The listing builds one solid part. Answer for the finished solid, in the listing's coordinates (mm). A direction names the side the tool comes from. Round coordinates to 2 decimals unless told otherwise and drop trailing zeros. Order: outer loops, then holes, each group sorted by start corner. A loop starts at its lowest first (then second) coordinate and runs counter-clockwise, first axis right, second up. Notation, with made-up numbers: (60, 32) - (70, 32) arc R9 cw to (70, 43) - close; hole circle Ø4 at (-21.75, 1). An arc over 180 degrees is marked (long way). One line per item, written item: value. Start each with the question number.
1. Flat-ended cylindrical pins translate along their axes: P1, Ø2, axis at x = 61.5, z = 25.5, coming from the +Y side; P2, Ø3, axis at x = 27.5, z = -29, coming from the -Y side; P3, Ø12, axis at x = 96.5, z = -0.5, coming from the +Y side; P4, Ø2.5, axis at x = 73, z = 32.689, coming from the -Y side. Find the tip coordinate at first contact, or state that the pin passes through.
2. Section D-D, the plane x = 109 is taken. Give the vertices of the cut face in (y, z), then the cut area to 3 significant figures.
3. Section C-C, the plane z = -16 is taken. Give the vertices of the cut face in (x, y), then the cut area to 3 significant figures.
4. A tool of negligible diameter and unlimited length cuts with its end or side. For faces 4 (the flat face through (44, -23, -7.451)), 5 (the flat face through (44, -25, 17.689)), 6 (the flat face through (63, -21, -10.131)), from which of +Z, -Z, +X, -X, +Y, -Y can it reach the whole face along a straight path? Write none if from no direction.
5. Section B-B, the plane x = 73 is taken. Count the separate pieces of the cut face and the enclosed holes in it, then the cut area to 3 significant figures.
6. Straight lines are drawn through the part: line 1 (Z direction, x = 73, y = -25); line 2 (X direction, y = -24, z = -31); line 3 (Z direction, x = 37, y = -4). For each, find the intervals that lie inside material, in ascending order.
7. For a pull along X with two mould halves and no side action, classify faces 1 (the flat face through (18, -3, -26)), 2 (the flat face through (97.72, -9.847, 20.896)), 3 (the cylindrical face through (62.86, -16.74, 20.36)) as released by +X, released by -X, zero draft, split by the parting line, or undercut.
Autodesk Inventor part; units mm, degrees
ref_plane "YZ Plane" through (0, 0, 0) normal (1, 0, 0) x (0, 1, 0)
ref_plane "XZ Plane" through (0, 0, 0) normal (0, 1, 0) x (-1, 0, 0)
ref_plane "XY Plane" through (0, 0, 0) normal (0, 0, 1) x (1, 0, 0)
ref_plane "Plan de construction16" through (10, -26.1714, -17.6889) normal (0, -1, 0) x (1, 0, 0)
sketch "Esquisse9" plane through (10, -26.1714, -17.6889) normal (0, -1, 0) x (1, 0, 0)
  line L0 (0, 35.3779) -> (8, 35.3779)
  line L1 (68, 1.8848) -> (68, 33.493)
  line L2 (0, 35.3779) -> (68, 35.3779)
  line L3 (68, 35.3779) -> (68, 32.0585)
  line L4 (0, 32.0585) -> (0, 35.3779)
  line L5 (0, 0) -> (8, 0)
  line L6 (0, 37.6889) -> (0, -2.3111)
  line L7 (68, 0) -> (0, 0)
  line L8 (0, 0) -> (0, 3.3237)
  line L9 (68, 3.3237) -> (68, 0)
  line L10 (68, 35.3779) -> (0, 35.3779)
  line L11 (0, 35.3779) -> (0, 0)
  line L12 (0, 0) -> (68, 0)
  line L13 (68, 0) -> (68, 35.3779)
  point P0 (-10, 17.6889)
  point P1 (67.75, 35.3779)
  point P2 (67.75, 0)
extrude "Extrusion11" add sketch "Esquisse9" against normal blind 3
ref_plane "Plan de construction18" through (78, -26.1714, -17.6889) normal (0, -1, 0) x (1, 0, 0)
sketch "Esquisse13" plane through (78, -26.1714, -17.6889) normal (0, -1, 0) x (1, 0, 0)
  line L0 (-65, 35.3779) -> (-60, 35.3779)
  line L1 (0, 35.3779) -> (-10, 35.3779)
  line L2 (-10, 35.3779) -> (-10, 55.3779)
  line L3 (-10, 55.3779) -> (0, 55.3779)
  line L4 (0, 55.3779) -> (0, 35.3779)
  line L5 (0, 35.3779) -> (0, 0) construction
  line L6 (0, 17.6889) -> (-68.1792, 17.6889) construction
  line L7 (-68.1792, 35.3779) -> (-58.1792, 35.3779)
  line L8 (-58.1792, 35.3779) -> (-58.1792, 55.3779)
  line L9 (-58.1792, 55.3779) -> (-68.1792, 55.3779)
  line L10 (-68.1792, 55.3779) -> (-68.1792, 35.3779)
  line L11 (-65, 0) -> (0, 0)
  line L12 (0, 0) -> (-10, 0)
  line L13 (-10, 0) -> (-10, -20)
  line L14 (-10, -20) -> (0, -20)
  line L15 (0, -20) -> (0, 0)
  line L16 (-68.1792, 0) -> (-58.1792, 0)
  line L17 (-58.1792, 0) -> (-58.1792, -20)
  line L18 (-58.1792, -20) -> (-68.1792, -20)
  line L19 (-68.1792, -20) -> (-68.1792, 0)
  line L20 (-5, 34.0863) -> (-5, 43.2092) construction
  circle A0 centre (-5, 50.3779) radius 2.25
  circle A1 centre (-63.1792, 50.3779) radius 2.25
  circle A2 centre (-63.1792, -15) radius 2.25
  line L21 (-5, -1.4113) -> (-5, -11.1612)
  circle A3 centre (-5, -15) radius 2.25
  point P0 (-78, 17.6889)
  point P1 (0, 1.8848)
  point P2 (0, 33.493)
  point P3 (-0.25, 35.3779)
  dimension "d45" = 10
  dimension "d46" = 20
  dimension "d47" = 10
  dimension "d48" = 20
  dimension "d49" = 4.5
  dimension "d50" = 4.5
  dimension "d51" = 4.5
  dimension "d52" = 4.5
  dimension "d57" = 0
  dimension "d58" = 5
  dimension "d59" = 5
  dimension "d60" = 5
  dimension "d61" = 5
extrude "Extrusion12" add sketch "Esquisse13" against normal blind 3
ref_plane "Plan de construction19" through (18, 0, 0) normal (1, 0, 0) x (0, 0, -1)
sketch "Esquisse14" plane through (18, 0, 0) normal (1, 0, 0) x (0, 0, -1)
  line L0 (-19.134, -23.1714) -> (-15.8041, -23.1714)
  line L1 (-19.134, -23.1714) -> (-15.8041, -23.1714)
  line L2 (-15.8041, -23.1714) -> (-36.599, 20)
  line L3 (-38.4838, 17) -> (-19.134, -23.1714)
  line L4 (-19.134, -23.1714) -> (-15.8041, -23.1714)
  line L5 (-19.134, -23.1714) -> (-15.8041, -23.1714)
  line L6 (-36.599, 20) -> (-38.4838, 17)
  line L7 (-15.8041, -23.1714) -> (-36.599, 20)
  line L8 (-36.599, 20) -> (-38.4838, 17)
  line L9 (-38.4838, 17) -> (-19.134, -23.1714)
  line L10 (-15.8041, -23.1714) -> (-36.599, 20)
  line L11 (-36.599, 20) -> (-38.4838, 17)
  line L12 (-38.4838, 17) -> (-19.134, -23.1714)
  line L13 (17.6889, -23.1714) -> (-17.6889, -23.1714)
  line L14 (-14.4365, -23.1714) -> (-35.9022, 21.1089)
  line L15 (-35.9022, 21.1089) -> (-36.599, 20)
  line L16 (0, 22.9524) -> (0, -23.1714) construction
  line L17 (15.8041, -23.1714) -> (36.599, 20)
  line L18 (-17.6889, -23.1714) -> (17.6889, -23.1714)
  line L19 (14.4365, -23.1714) -> (35.9022, 21.1089)
  line L20 (35.9022, 21.1089) -> (36.599, 20)
  line L21 (14.4365, -23.1714) -> (15.8041, -23.1714)
  line L22 (35.9022, 21.1089) -> (36.599, 20)
  line L23 (15.8041, -23.1714) -> (36.599, 20)
  line L24 (35.9022, 21.1089) -> (14.4365, -23.1714)
  line L25 (-36.599, 20) -> (-37.5414, 18.5)
  line L26 (-17.6889, -23.1714) -> (-17.6889, -26.1714)
  line L27 (-37.5414, 18.5) -> (-17.6889, -23.1714)
  line L28 (-17.6889, -23.1714) -> (-14.4365, -23.1714)
  line L29 (35.9022, 21.1089) -> (37.5414, 18.5)
  line L30 (37.5414, 18.5) -> (17.4582, -23.1714)
  line L31 (14.4365, -23.1714) -> (17.4582, -23.1714)
  point P0 (0, 0)
ref_plane "Plan de construction10" through (78, -23.1714, 15.8041) normal (0, 1, 0) x (1, 0, 0)
sketch "Esquisse15" plane through (78, -23.1714, 15.8041) normal (0, 1, 0) x (1, 0, 0)
  line L0 (0, 53.493) -> (0, -21.8848)
  line L1 (-68, 5.6727) -> (0, 5.6727)
  line L2 (0, 5.6727) -> (0, 8.3531)
  line L3 (0, 8.3531) -> (-68, 8.3531)
  line L4 (-68, 8.3531) -> (-68, 5.6727)
  line L5 (-68, 33.493) -> (-68, -1.8848)
  line L6 (-68, -1.8848) -> (-68, 33.493) construction
  line L7 (-68, 15.8041) -> (0, 15.8041) construction
  line L8 (0, 53.493) -> (0, -21.8848)
  line L9 (-68, 25.9355) -> (0, 25.9355)
  line L10 (0, 25.9355) -> (0, 23.255)
  line L11 (0, 23.255) -> (-68, 23.255)
  line L12 (-68, 23.255) -> (-68, 25.9355)
  line L13 (-68, -1.8848) -> (-68, 33.493)
  line L14 (-68, 33.493) -> (-68, -1.8848) construction
  point P0 (-78, 15.8041)
extrude "Extrusion14" add sketch "Esquisse15" along normal blind 4 contours L0 L11 L5 L9 | L0 L1 L4 L3
ref_plane "Plan de construction11" through (68, -26.1714, -37.6889) normal (0, -1, 0) x (1, 0, 0)
sketch "Esquisse16" plane through (68, -26.1714, -37.6889) normal (0, -1, 0) x (1, 0, 0)
  line L0 (-58, 45.1399) -> (10, 45.1399)
  line L1 (-58, 30.238) -> (10, 30.238)
  line L2 (3.117, 45.1399) -> (-52.8886, 45.1399)
  line L3 (-52.8886, 45.1399) -> (-52.8886, 30.238)
  line L4 (-52.8886, 30.238) -> (3.117, 30.238)
  line L5 (3.117, 30.238) -> (3.117, 45.1399)
  point P0 (-68, 37.6889)
extrude "Extrusion15" cut sketch "Esquisse16" against normal blind 4
extrude "Extrusion16" add sketch "Esquisse14" along normal up to surface (60 mm away) contours L19 L20 L17 L13 | L27 L6 L2 L0 | L2 L15 L14 L13 | L17 L29 L30 L13
ref_plane "Plan de construction20" through (18, 21.1089, -35.9022) normal (0, -1, 0) x (1, 0, 0)
sketch "Esquisse17" plane through (18, 21.1089, -35.9022) normal (0, -1, 0) x (1, 0, 0)
  circle A0 centre (18.615, 35.9022) radius 22.5 construction
  circle A1 centre (45.1277, 16.765) radius 1.25
  line L0 (50, 53.5912) -> (50, 73.5912)
  circle A2 centre (13.6149, 6.5446) radius 1.25
  line L1 (60, 43.3532) -> (60, 28.4513)
  line L2 (-11.4468, 35.9022) -> (31.8074, 35.9022) construction
  circle A3 centre (45.1277, 55.0395) radius 1.25
  line L3 (13.6149, 53.5912) -> (50, -1.7867)
  circle A4 centre (13.6149, 65.2599) radius 1.25
  point P0 (-18, 35.9022)
  dimension "d68" = 45
  dimension "d69" = 2.5
  dimension "d70" = 2.5
  dimension "d71" = 41.385
extrude "Extrusion17" cut sketch "Esquisse17" along normal up to surface (44.2803 mm away)
sketch "Esquisse18" plane through (18, 21.1089, -35.9022) normal (0, -1, 0) x (1, 0, 0)
  line L0 (-5.0895, 79.4289) -> (61.3071, 79.4289)
  line L1 (61.3071, 79.4289) -> (61.3071, 14.8125)
  line L2 (61.3071, 14.8125) -> (-5.0895, 14.8125)
  line L3 (-5.0895, 14.8125) -> (-5.0895, 79.4289)
  point P0 (-18, 35.9022)
extrude "Extrusion18" cut sketch "Esquisse18" along normal blind 18
sketch "Esquisse19" plane through (78, -26.1714, 37.6889) normal (1, 0, 0) x (0, 0, -1)
  line L0 (10.5125, 29.2803) -> (7.4799, 29.2803)
  line L1 (20, 3) -> (7.4799, 29.2803)
  line L2 (0, 3) -> (20, 3)
  line L3 (0, 0) -> (0, 3)
  line L4 (75.3779, 0) -> (0, 0)
  line L5 (75.3779, 0) -> (75.3779, 3)
  line L6 (55.1472, 3) -> (75.3779, 3)
  line L7 (75.2303, 44.6714) -> (55.1472, 3)
  line L8 (73.5912, 47.2803) -> (75.2303, 44.6714)
  line L9 (52.1254, 3) -> (73.5912, 47.2803)
  line L10 (47.8203, 3) -> (52.1254, 3)
  line L11 (47.8203, 3) -> (47.8203, 7)
  line L12 (45.1399, 7) -> (47.8203, 7)
  line L13 (45.1399, 3) -> (45.1399, 7)
  line L14 (30.238, 3) -> (45.1399, 3)
  line L15 (30.238, 3) -> (30.238, 7)
  line L16 (27.5576, 7) -> (30.238, 7)
  line L17 (27.5576, 3) -> (27.5576, 7)
  line L18 (23.2524, 3) -> (27.5576, 3)
  line L19 (10.5125, 29.2803) -> (23.2524, 3)
  line L20 (0, 3) -> (20, 3)
  line L21 (20, 3) -> (20, 0)
  line L22 (20, 0) -> (55.3779, 0)
  line L23 (55.1472, 3) -> (75.2303, 44.6714)
  line L24 (47.8203, 0) -> (50.6711, 0)
  line L25 (20, 3) -> (20, 0)
  line L26 (20, 0) -> (55.1472, 0)
  line L27 (55.1472, 3) -> (55.1472, 0)
  line L28 (55.1472, 3) -> (75.2303, 44.6714)
  point P0 (37.6889, 26.1714)
extrude "Extrusion19" add sketch "Esquisse19" along normal blind 40 contours L19 L18 L17 L16 L15 L14 L13 L12 L11 L10 L9 L8 L7 L27 L4 L21 L1 L0
properties part number "new_cuiller"
Answer list:
1. P1: stops at y = 1.71
1. P2: stops at y = -2.34
1. P3: stops at y = -23.17
1. P4: passes through
2. outline: (-26.17, -17.46) - (-23.17, -17.46) - (18.5, -37.54) - (21.11, -35.9) - (-23.17, -14.44) - (-23.17, -10.13) - (-19.17, -10.13) - (-19.17, -7.45) - (-23.17, -7.45) - (-23.17, 7.45) - (-19.17, 7.45) - (-19.17, 10.13) - (-23.17, 10.13) - (-23.17, 14.44) - (3.11, 27.18) - (3.11, 30.21) - (-23.17, 17.69) - (-26.17, 17.69) - close
2. area: 337 mm²
3. outline: (10, -26.17) - (118, -26.17) - (118, -19.95) - (18, -19.95) - (18, -23.17) - (10, -23.17) - close
3. area: 647 mm²
4. face 4: +Y
4. face 5: +Z, -Y
4. face 6: +X, -X, +Y
5. separate pieces: 3
5. enclosed holes: 0
5. area: 430 mm²
6. line 1: z = -37.69 to -34.94, -30.44 to 30.44, 34.94 to 37.69
6. line 2: x = 9.82 to 13.33, 16.31 to 19.82, 68 to 71.51, 74.49 to 78
6. line 3: z = -26.7 to -23.73, 23.73 to 26.82
7. face 1: released by -X
7. face 2: zero draft
7. face 3: undercut
